from build123d import *

# Parameters (mm, degrees)
SKETCH_1_R      = 3.4
SKETCH_1_R_2    = 2.5
EXTRUDE_1_DEPTH = 1000


with BuildPart() as part:
    # Эскиз1 → Бобышка-Вытянуть1 (new body)
    with BuildSketch(Plane.XY):
        with BuildLine():
            Line((-10, 20), (-20, 20))
            Line((-20, 20), (-20, 6.3))
            ThreePointArc((-20, 6.3), (-19.912132034, 6.087867966), (-19.7, 6))
            Line((-19.7, 6), (-19, 6))
            Line((-19, 6), (-19, 5.3))
            ThreePointArc((-19, 5.3), (-18.912132034, 5.087867966), (-18.7, 5))
            Line((-18.7, 5), (-15.8, 5))
            ThreePointArc((-15.8, 5), (-15.587867966, 5.087867966), (-15.5, 5.3))
            Line((-15.5, 5.3), (-15.5, 8))
            Line((-15.5, 8), (-16.7, 8))
            ThreePointArc((-16.7, 8), (-16.912132034, 8.087867966), (-17, 8.3))
            Line((-17, 8.3), (-17, 10.1))
            ThreePointArc((-17, 10.1), (-16.912132034, 10.312132034), (-16.7, 10.4))
            Line((-16.7, 10.4), (-12.7, 10.4))
            Line((-12.7, 10.4), (-6, 3.7))
            Line((-6, 3.7), (-6, -3.7))
            Line((-6, -3.7), (-9.9, -7.6))
            Line((-9.9, -7.6), (-15.2, -7.6))
            ThreePointArc((-15.2, -7.6), (-15.412132034, -7.512132034), (-15.5, -7.3))
            Line((-15.5, -7.3), (-15.5, -4.3))
            ThreePointArc((-15.5, -4.3), (-15.587867966, -4.087867966), (-15.8, -4))
            Line((-15.8, -4), (-18.7, -4))
            ThreePointArc((-18.7, -4), (-18.912132034, -4.087867966), (-19, -4.3))
            Line((-19, -4.3), (-19, -5))
            Line((-19, -5), (-19.7, -5))
            ThreePointArc((-19.7, -5), (-19.912132034, -5.087867966), (-20, -5.3))
            Line((-20, -5.3), (-20, -10))
            Line((-20, -10), (-5.4, -10))
            ThreePointArc((-5.4, -10), (-5.187867966, -9.912132034), (-5.1, -9.7))
            Line((-5.1, -9.7), (-5.1, -9))
            Line((-5.1, -9), (-4.4, -9))
            ThreePointArc((-4.4, -9), (-4.187867966, -8.912132034), (-4.1, -8.7))
            Line((-4.1, -8.7), (-4.1, -6))
            Line((-4.1, -6), (4.1, -6))
            Line((4.1, -6), (4.1, -8.7))
            ThreePointArc((4.1, -8.7), (4.187867966, -8.912132034), (4.4, -9))
            Line((4.4, -9), (5.1, -9))
            Line((5.1, -9), (5.1, -9.7))
            ThreePointArc((5.1, -9.7), (5.187867966, -9.912132034), (5.4, -10))
            Line((5.4, -10), (20, -10))
            Line((20, -10), (20, -5.3))
            ThreePointArc((20, -5.3), (19.912132034, -5.087867966), (19.7, -5))
            Line((19.7, -5), (19, -5))
            Line((19, -5), (19, -4.3))
            ThreePointArc((19, -4.3), (18.912132034, -4.087867966), (18.7, -4))
            Line((18.7, -4), (15.8, -4))
            ThreePointArc((15.8, -4), (15.587867966, -4.087867966), (15.5, -4.3))
            Line((15.5, -4.3), (15.5, -7.3))
            ThreePointArc((15.5, -7.3), (15.412132034, -7.512132034), (15.2, -7.6))
            Line((15.2, -7.6), (9.9, -7.6))
            Line((9.9, -7.6), (6, -3.7))
            Line((6, -3.7), (6, 3.7))
            Line((6, 3.7), (12.7, 10.4))
            Line((12.7, 10.4), (16.7, 10.4))
            ThreePointArc((16.7, 10.4), (16.912132034, 10.312132034), (17, 10.1))
            Line((17, 10.1), (17, 8.3))
            ThreePointArc((17, 8.3), (16.912132034, 8.087867966), (16.7, 8))
            Line((16.7, 8), (15.5, 8))
            Line((15.5, 8), (15.5, 5.3))
            ThreePointArc((15.5, 5.3), (15.587867966, 5.087867966), (15.8, 5))
            Line((15.8, 5), (18.7, 5))
            ThreePointArc((18.7, 5), (18.912132034, 5.087867966), (19, 5.3))
            Line((19, 5.3), (19, 6))
            Line((19, 6), (19.7, 6))
            ThreePointArc((19.7, 6), (19.912132034, 6.087867966), (20, 6.3))
            Line((20, 6.3), (20, 20))
            Line((20, 20), (10, 20))
            Line((10, 20), (5.7, 20))
            ThreePointArc((5.7, 20), (5.487867966, 19.912132034), (5.4, 19.7))
            Line((5.4, 19.7), (5.4, 19))
            Line((5.4, 19), (4.4, 19))
            ThreePointArc((4.4, 19), (4.187867966, 18.912132034), (4.1, 18.7))
            Line((4.1, 18.7), (4.1, 15.8))
            ThreePointArc((4.1, 15.8), (4.187867966, 15.587867966), (4.4, 15.5))
            Line((4.4, 15.5), (9.7, 15.5))
            ThreePointArc((9.7, 15.5), (9.912132034, 15.412132034), (10, 15.2))
            Line((10, 15.2), (10, 12))
            Line((10, 12), (4, 6))
            Line((4, 6), (-4, 6))
            Line((-4, 6), (-10, 12))
            Line((-10, 12), (-10, 15.2))
            ThreePointArc((-10, 15.2), (-9.912132034, 15.412132034), (-9.7, 15.5))
            Line((-9.7, 15.5), (-4.4, 15.5))
            ThreePointArc((-4.4, 15.5), (-4.187867966, 15.587867966), (-4.1, 15.8))
            Line((-4.1, 15.8), (-4.1, 18.7))
            ThreePointArc((-4.1, 18.7), (-4.187867966, 18.912132034), (-4.4, 19))
            Line((-4.4, 19), (-5.4, 19))
            Line((-5.4, 19), (-5.4, 19.7))
            ThreePointArc((-5.4, 19.7), (-5.487867966, 19.912132034), (-5.7, 20))
            Line((-5.7, 20), (-10, 20))
        make_face()
        Circle(SKETCH_1_R, mode=Mode.SUBTRACT)
        with Locations((15, 15)):
            Circle(SKETCH_1_R_2, mode=Mode.SUBTRACT)
        with Locations((-15, 15)):
            Circle(SKETCH_1_R_2, mode=Mode.SUBTRACT)
    extrude(amount=EXTRUDE_1_DEPTH)


solid = part.part
The listing builds one solid part. Answer for the finished solid, in the listing's coordinates (mm). Give positions to 0.01 mm unless a question says otherwise; leave off trailing zeros. One line per question, with ' | ' between items. Start each with the question number.
1. Given pin 1 Ø0.5 at (x, z) = (4.5, 335.5) entering from +Y; pin 2 Ø0.6 at (y, z) = (-4.5, 394) entering from -X; pin 3 Ø3 at (x, y) = (1, 16.5) entering from +Z, each flat-ended and moving along its own axis, determine where each tip first touches the part or whether it passes through.
2. Section A-A (z = 905) is taken. State how many separate pieces and enclosed holes the cut face has, plus the area to 3 significant figures.
3. Find the intervals of material crossed by probe 1 along Y at (x, z) = (-15, 366); probe 2 along X at (y, z) = (14.75, 262.5); probe 3 along Y at (x, z) = (14.5, 665.5), in increasing order.
Response values:
1) pin 1: y = 19 | pin 2: x = -19 | pin 3: through
2) separate pieces: 1 | enclosed holes: 3 | area: 522 mm2
3) probe 1: -10 to -7.6, 10.4 to 12.5, 17.5 to 20 | probe 2: -20 to -17.49, -12.51 to -10, 10 to 12.51, 17.49 to 20 | probe 3: -10 to -7.6, 10.4 to 12.55, 17.45 to 20
